```python
from build123d import *

# Parameters (mm, degrees)
SKETCH1_R           = 30
SKETCH1_W           = 150
SKETCH1_H           = 40
BOSS_EXTRUDE1_DEPTH = 30
SKETCH2_R           = 15
CUT_EXTRUDE1_DEPTH  = 8.9


with BuildPart() as part:
    # Sketch1 → Boss-Extrude1 (new body)
    with BuildSketch(Plane.XY):
        Circle(SKETCH1_R)
        with Locations((150, 0)):
            Circle(SKETCH1_R)
        with Locations((75, 0)):
            Rectangle(SKETCH1_W, SKETCH1_H)
    extrude(amount=BOSS_EXTRUDE1_DEPTH)

    # Sketch2 → Cut-Extrude1 (cut)
    with BuildSketch(Plane.XY.offset(30)):
        Circle(SKETCH2_R)
    extrude(amount=-CUT_EXTRUDE1_DEPTH, mode=Mode.SUBTRACT)


solid = part.part
```
Source: CAD feature listing. Evaluate the final solid. Frame: model axes, mm. A direction names the side the tool comes from. Round coordinates to 2 decimals unless told otherwise and drop trailing zeros. Loops run counter-clockwise (first coordinate to the right, second up) from the corner with the lowest first, then second, coordinate; pieces in that order, holes last. Notation, with made-up numbers: M -38.5,74 L -8.5,74 A23 ccw -8.5,96 Z; hole C 49,-6.5 d11. An arc over 180 degrees is marked long. Put each result on its own line as item: value.
(1) Pull-direction query (X, two-part tool) for faces 6 (the face through (-29.983, 1.013, 14.79)), 7 (the face through (-14.985, 0.66, 25.612)), 8 (the face through (74, 0, 30)); classes: released by +X, released by -X, zero draft, split by the parting line, or undercut.
Solutions:
face 6: undercut
face 7: undercut
face 8: zero draft
(2) Access query for faces 1 (the face through (0, 0, 21.1)), 2 (the face through (74, -20, 15)), 3 (the face through (179.983, -1.013, 14.79)), 4 (the face through (74, 0, 0)), 5 (the face through (74, 20, 15)). Directions: +Z, -Z, +X, -X, +Y, -Y. A direction counts if a zero-diameter tool reaches every point of the face in a straight line with its end or side. Return the directions, or none.
Solutions:
face 1: +Z
face 2: +Z, -Z, -Y
face 3: +Z, -Z
face 4: -Z, +X, -X, +Y, -Y
face 5: +Z, -Z, +Y
(3) Section D-D, the plane z = 12.25. Return loops of the section in (x, y), and give its area (3 significant figures).
Solutions:
outline: M 22.36,-20 L 127.64,-20 A30 ccw long 127.64,20 L 22.36,20 A30 ccw long Z
area: 9,450 mm²
(4) First-contact query: pin 1 (5 mm diameter, centred on y = -15.5, z = 22, fed in from -X); pin 2 (10 mm diameter, centred on x = 107, z = 23, fed in from +Y); pin 3 (5 mm diameter, centred on y = 14.5, z = 15, fed in from +X). Flat tips, straight axial feed; report the tip coordinate or a pass-through.
Solutions:
pin 1: x = -27.04
pin 2: y = 20
pin 3: x = 177.5
(5) Ray query, line 1 (Y direction, x = 0, z = 24.5); line 2 (Y direction, x = 113, z = 4.75); line 3 (Y direction, x = -12, z = 24.75). Return the intervals inside material, ascending. Write a range as [from, to].
Solutions:
line 1: [-30, -15], [15, 30]
line 2: [-20, 20]
line 3: [-27.5, -9], [9, 27.5]
(6) Section A-A, the plane y = 0. Return loops of the section in (x, z).
Solutions:
outline: M -30,0 L 180,0 L 180,30 L 15,30 L 15,21.1 L -15,21.1 L -15,30 L -30,30 Z
(7) Section B-B, the plane y = -25. Return loops of the section in (x, z), and give its area (3 significant figures).
Solutions:
outline: M -16.58,0 L 16.58,0 L 16.58,30 L -16.58,30 Z; M 133.42,0 L 166.58,0 L 166.58,30 L 133.42,30 Z
area: 1,990 mm²
(8) Section C-C, the plane x = 0. Return loops of the section in (y, z), and give its area (3 significant figures).
Solutions:
outline: M -30,0 L 30,0 L 30,30 L 15,30 L 15,21.1 L -15,21.1 L -15,30 L -30,30 Z
area: 1,530 mm²
